Part model, mm, in its own coordinate system. A direction names the side the tool comes from. Round coordinates to 2 decimals unless told otherwise and drop trailing zeros. Write each loop counter-clockwise with the first axis right and the second up, starting at its lowest first coordinate (ties: lowest second). Pieces come first, ordered by that corner, then holes. Notation, with made-up numbers: (-7.5, 6) -> (33.5, 6) arc R7 ccw to (33.5, 19) -> close; hole circle Ø3 at (46.5, 67.5). An arc over 180 degrees is marked (long way). Return JSON: item names as keys, results as strings. Group by question number.
(1) Mould opens along X. For faces 4 (the cylindrical face through (-4.425, 8.986, 6.386)), 5 (the flat face through (0, 4, 5)), 6 (the cylindrical face through (15.575, 8.986, 6.386)), 7 (the flat face through (1, 6, 0)) say: +X half, -X half, draft (parallel to the pull), parting line (faces both ways), or undercut.
(2) Drill centre lines: L1, parallel to X at y = 9.25, z = 5; L2, parallel to X at y = 9.25, z = 7.5; L3, parallel to X at y = 5.25, z = 9.25. Where is each one in solid material? Low to high. Write a range as from..to.
(3) Saw through at B-B (z = 5). List the corners of the cut face in (x, y).
(4) Saw through at D-D (y = 4.25). List the corners of the cut face in (x, z), plus the area to 3 significant figures.
(5) Saw through at A-A (y = 9). List the corners of the cut face in (x, z).
(6) Tool access for faces 1 (the flat face through (2, 6, 5)), 2 (the flat face through (13.8, 8, 3.8)), 3 (the flat face through (-3.8, 8, 3.8)): list every direction of +Z, -Z, +X, -X, +Y, -Y with a clear straight run to the whole face (end or side of a thin tool).
(7) Drop flat-ended pins along their axis: pin 1 Ø4 at (x, y) = (13.5, 3) entering from +Z; pin 2 Ø4 at (y, z) = (2.5, 5) entering from +X; pin 3 Ø2.5 at (y, z) = (4.5, 4) entering from -X; pin 4 Ø5 at (x, z) = (14, 6) entering from -Y. Give the stop position or say it passes through.
(8) Saw through at C-C (x = 15). List the corners of the cut face in (y, z).
Autodesk Inventor part; units mm, degrees
ref_plane "YZ Plane" through (0, 0, 0) normal (1, 0, 0) x (0, 1, 0)
ref_plane "XZ Plane" through (0, 0, 0) normal (0, 1, 0) x (-1, 0, 0)
ref_plane "XY Plane" through (0, 0, 0) normal (0, 0, 1) x (1, 0, 0)
sketch "Sketch1" plane through (0, 0, 0) normal (0, 0, 1) x (1, 0, 0)
  line L0 (0, 0) -> (10, 0)
  line L1 (10, 0) -> (10, 8)
  line L2 (0, 8) -> (0, 0)
  line L3 (8, 10) -> (8, 2)
  line L4 (8, 2) -> (2, 2)
  line L5 (2, 2) -> (2, 8)
  line L6 (0, 8) -> (-10, 8)
  line L7 (-10, 8) -> (-10, 10)
  line L8 (10, 8) -> (20, 8)
  line L9 (20, 8) -> (20, 10)
  line L10 (2, 8) -> (2, 10)
  line L11 (-10, 10) -> (2, 10)
  line L12 (8, 10) -> (20, 10)
  line L13 (10, 10) -> (8, 10)
  line L14 (2, 10) -> (0, 10)
  dimension "d3" = 10
  dimension "d4" = 10
extrude "Extrusion1" add sketch "Sketch1" along normal blind 10
sketch "Sketch2" plane through (-10, 10, 0) normal (0, 1, 0) x (1, 0, 0)
  line L0 (12, -10) -> (0, -10)
  line L1 (0, 0) -> (0, -10)
  line L2 (30, 0) -> (18, 0)
  line L3 (30, 0) -> (30, -10)
  point P0 (10, 0)
  point P1 (5, -5)
  point P2 (25, -5)
  dimension "d14" = 5
  dimension "d15" = 5
  dimension "d16" = 5
  dimension "d17" = 5
hole "Hole1" at (-5, 10, 5) at (15, 10, 5) direction (0, -1, 0) diameter 3 end through all
properties part number "CAM_HOLD"
Computed values:
{
 "1": {"face 4": "undercut", "face 5": "-X half", "face 6": "undercut", "face 7": "draft"},
 "2": {"L1": "-10..-6.5, -3.5..2, 8..13.5, 16.5..20", "L2": "-10..2, 8..20", "L3": "0..2, 8..10"},
 "3": {"outline": "(-10, 8) -> (-6.5, 8) -> (-6.5, 10) -> (-10, 10) -> close; (-3.5, 8) -> (0, 8) -> (0, 0) -> (10, 0) -> (10, 8) -> (13.5, 8) -> (13.5, 10) -> (8, 10) -> (8, 2) -> (2, 2) -> (2, 10) -> (-3.5, 10) -> close; (16.5, 8) -> (20, 8) -> (20, 10) -> (16.5, 10) -> close"},
 "4": {"outline": "(0, 0) -> (2, 0) -> (2, 10) -> (0, 10) -> close; (8, 0) -> (10, 0) -> (10, 10) -> (8, 10) -> close", "area": "40.0 mm2"},
 "5": {"outline": "(-10, 0) -> (2, 0) -> (2, 10) -> (-10, 10) -> close; (8, 0) -> (20, 0) -> (20, 10) -> (8, 10) -> close; hole circle Ø3 at (-5, 5); hole circle Ø3 at (15, 5)"},
 "6": {"face 1": "+Z, -Z, +Y", "face 2": "+Z, -Z, +X, -Y", "face 3": "+Z, -Z, -X, -Y"},
 "7": {"pin 1": "through", "pin 2": "x = 10", "pin 3": "x = 0", "pin 4": "y = 8"},
 "8": {"outline": "(8, 0) -> (10, 0) -> (10, 3.5) -> (8, 3.5) -> close; (8, 6.5) -> (10, 6.5) -> (10, 10) -> (8, 10) -> close"}
}
